CAD build for the part. Positions are in the model's coordinates, mm. A direction names the side the tool comes from. Round coordinates to 2 decimals unless told otherwise and drop trailing zeros. Loops run counter-clockwise (first coordinate to the right, second up) from the corner with the lowest first, then second, coordinate; pieces in that order, holes last. Notation, with made-up numbers: (19, 60.5) -> (52, 60.5) arc R18 cw to (52, 76.5) -> close; hole circle Ø5 at (5, 1.5). An arc over 180 degrees is marked (long way). Answer as CSV lines item,"result".
```python
from build123d import *

# Parameters (mm, degrees)
CUT_EXTRUDE_1_DEPTH = 2
FILLET_1_R          = 0.3
CHAMFER_1_SIZE      = 0.3


with BuildPart() as part:
    # Эскиз1 → Повернуть1 (revolve)
    with BuildSketch(Plane(origin=(0, 0, 0), x_dir=(0, 0, -1), z_dir=(1, 0, 0)), mode=Mode.PRIVATE) as revolve_1_sk:
        Polygon((0, 0), (0, 2.5), (3, 2.5), (3, 1.5), (11, 1.5), (11, 0), align=None)
    revolve(revolve_1_sk.sketch.rotate(Axis((0, 0, 0), (0, 0, 1)), 90), axis=Axis((0, 0, 0), (0, 0, 1)))

    # Эскиз2 → Вырез-Вытянуть1 (cut)
    with BuildSketch(Plane.XY):
        Polygon((1.443375673, 0), (0.721687836, 1.25), (-0.721687836, 1.25), (-1.443375673, 0), (-0.721687836, -1.25), (0.721687836, -1.25), align=None)
    extrude(amount=-CUT_EXTRUDE_1_DEPTH, mode=Mode.SUBTRACT)

    # Скругление1
    fillet_1_edges = [part.edges().sort_by_distance(p)[0] for p in [
        (1.5, 0, -3),
    ]]
    fillet(fillet_1_edges, radius=FILLET_1_R)

    # Фаска1
    chamfer_1_edges = [part.edges().sort_by_distance(p)[0] for p in [
        (1.5, 0, -11),
    ]]
    chamfer(chamfer_1_edges, length=CHAMFER_1_SIZE)


solid = part.part
```
Q1. Slice it at C-C, the plane z = -9. Give the cut face in (x, y).
Results:
outline,"circle Ø3 at (0, 0)"
Q2. Drop flat-ended pins along their axis: pin 1 Ø1 at (y, z) = (0.5, -5) entering from -X; pin 2 Ø1 at (x, z) = (0.5, -5) entering from -Y; pin 3 Ø2 at (x, z) = (0, -10) entering from +Y. Give the stop position or say it passes through.
Results:
pin 1,"x = -1.5"
pin 2,"y = -1.5"
pin 3,"y = 1.5"
Q3. Slice it at A-A, the plane z = -1.5. Give the cut face in (x, y), and give its area (3 significant figures).
Results:
outline,"circle Ø5 at (0, 0); hole (-1.44, 0) -> (-0.72, -1.25) -> (0.72, -1.25) -> (1.44, 0) -> (0.72, 1.25) -> (-0.72, 1.25) -> close"
area,"14.2 mm2"
Q4. Two-plate mould, pull along Y, no slides. Class faces 1 (the flat face through (0, 1.25, -1)), 2 (the flat face through (1.1, 1.1, 0)), 3 (the cylindrical face through (-1.43, -0.45, -7.05)): pulls with the +Y half, pulls with the -Y half, needs draft (parallel to the pull), parting line crosses it, or undercut.
Results:
face 1,"undercut"
face 2,"needs draft"
face 3,"parting line crosses it"
Q5. Tool access for faces 4 (the flat face through (-1.08, 0.63, -0.99)), 5 (the flat face through (0, 0, -11)), 6 (the flat face through (1, -2, -3)): list every direction of +Z, -Z, +X, -X, +Y, -Y with a clear straight run to the whole face (end or side of a thin tool).
Results:
face 4,"+Z"
face 5,"-Z, +X, -X, +Y, -Y"
face 6,"-Z"
Q6. Probe L1, parallel to Y at x = 0, z = -0.5; L2, parallel to Y at x = -0.55, z = -1.5; L3, parallel to Z at x = 1.6, y = 0.85. List the from-to ranges inside material, lowest first. Write a range as [from, to].
Results:
L1,"[-2.5, -1.25], [1.25, 2.5]"
L2,"[-2.44, -1.25], [1.25, 2.44]"
L3,"[-3, 0]"
Q7. Slice it at B-B, the plane x = 0. Give the cut face in (y, z), and give its area (3 significant figures).
Results:
outline,"(-2.5, -3) -> (-1.8, -3) arc R0.3 cw to (-1.5, -3.3) -> (-1.5, -10.7) -> (-1.2, -11) -> (1.2, -11) -> (1.5, -10.7) -> (1.5, -3.3) arc R0.3 cw to (1.8, -3) -> (2.5, -3) -> (2.5, 0) -> (1.25, 0) -> (1.25, -2) -> (-1.25, -2) -> (-1.25, 0) -> (-2.5, 0) -> close"
area,"33.9 mm2"
